Input: dimensioned drawing with shaded views. Units: mm. Origin: part minimum x, y, z. Round coordinates to 2 decimals unless told otherwise and drop trailing zeros. Loops run counter-clockwise (first coordinate to the right, second up) from the corner with the lowest first, then second, coordinate; pieces in that order, holes last. Notation, with made-up numbers: M -26,13 L 7,13 A30 cw 7,50 Z; hole C -27.75,-23 d8. An arc over 180 degrees is marked long. Write each question's results on one line, items separated by ' | '. Start each with the question number.
1. Section A-A on x = 356. Output: boundary loops of the cut face in (y, z).
2. Ray query, line 1 (X direction, y = 34, z = 345.5) (1 decimal); line 2 (X direction, y = 7, z = 35.5); line 3 (X direction, y = 27, z = 94.5). Return the intervals inside material, ascending.
3. Section B-B on y = 18. Output: boundary loops of the cut face in (x, z) (1 decimal).
4. Contact query for flat-ended pins moving along their axis: pin 1 Ø3 at (y, z) = (18.5, 138) entering from +X; pin 2 Ø6 at (y, z) = (6, 251) entering from +X; pin 3 Ø1.5 at (y, z) = (15.5, 190.5) entering from +X. Output: stop coordinate, or through.
5. Section C-C on z = 174. Output: boundary loops of the cut face in (x, y).
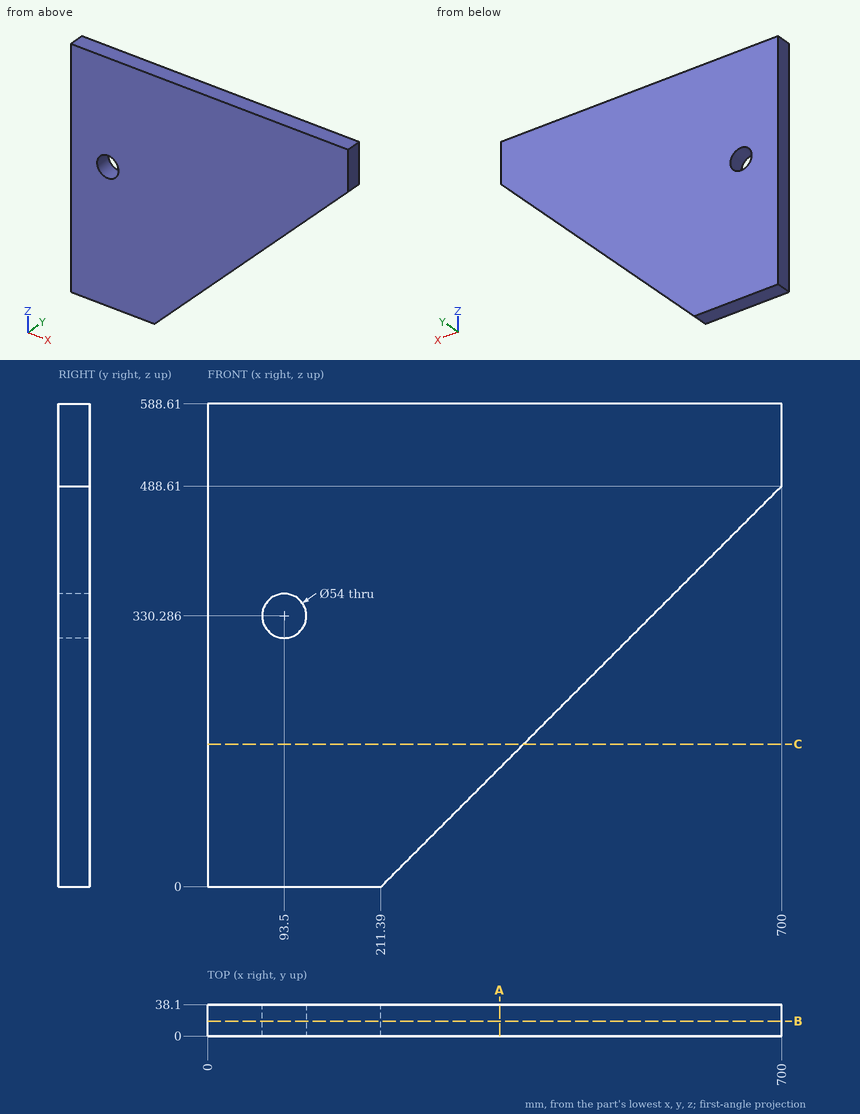
Taken from the geometry:
1) outline: M 0,144.61 L 38.1,144.61 L 38.1,588.61 L 0,588.61 Z
2) line 1: 0 to 71.2, 115.8 to 556.9 | line 2: 0 to 246.89 | line 3: 0 to 305.89
3) outline: M 0,0 L 211.4,0 L 700,488.6 L 700,588.6 L 0,588.6 Z; hole C 93.5,330.3 d54
4) pin 1: x = 350.89 | pin 2: x = 465.39 | pin 3: x = 402.64
5) outline: M 0,0 L 385.39,0 L 385.39,38.1 L 0,38.1 Z
